The model under review builds one solid part; all positions refer to its coordinate system, in mm. A direction names the side the tool comes from. Coordinates: 2 decimals unless noted, no trailing zeros. Loops run counter-clockwise (first coordinate to the right, second up) from the corner with the lowest first, then second, coordinate; pieces in that order, holes last. Notation, with made-up numbers: M -38.5,65 L 8.5,65 A17 ccw 8.5,80 Z; hole C 11.5,38.25 d1. An arc over 180 degrees is marked long. Use one line per item in the form item = value.
```python
from build123d import *

# Parameters (mm, degrees)
F0_W     = 20
F0_H     = 20
F1_DEPTH = 100
F2_R     = 5
F3_DEPTH = 20.001
F4_R     = 5
F5_DEPTH = 20.001
F6_W     = 22
F6_H     = 20
F6_R     = 5
F7_DEPTH = 10
F8_W     = 30
F8_H     = 20
F8_R     = 5
F9_DEPTH = 10
F10_R    = 9.99999


# Not quite as in the source:
# - a fillet or chamfer is up to 0.001 mm smaller than in the source, because OpenCascade refuses the exact size


with BuildPart() as f1:
    # F0 (on Front) → F1 (new body)
    with BuildSketch(Plane.XZ):
        Rectangle(F0_W, F0_H)
    extrude(amount=F1_DEPTH)

    # F2 (on face) → F3 (cut, through all)
    with BuildSketch(Plane.YZ.offset(10)):
        with Locations((-90, 0)):
            Circle(F2_R)
    extrude(amount=-F3_DEPTH, mode=Mode.SUBTRACT)

    # F4 (on face) → F5 (cut, through all)
    with BuildSketch(Plane.YZ.offset(10)):
        with Locations((-10, 0)):
            Circle(F4_R)
    extrude(amount=-F5_DEPTH, mode=Mode.SUBTRACT)

    # F6 (on face) → F7 (cut)
    with BuildSketch(Plane.YZ.offset(10)):
        with Locations((-11, 0)):
            Rectangle(F6_W, F6_H)
        with Locations((-10, 0)):
            Circle(F6_R, mode=Mode.SUBTRACT)
    extrude(amount=-F7_DEPTH, mode=Mode.SUBTRACT)

    # F8 (on face) → F9 (cut)
    with BuildSketch(Plane(origin=(-10, 0, 0), x_dir=(0, -1, 0), z_dir=(-1, 0, 0))):
        with Locations((85, 0)):
            Rectangle(F8_W, F8_H)
        with Locations((90, 0)):
            Circle(F8_R, mode=Mode.SUBTRACT)
    extrude(amount=-F9_DEPTH, mode=Mode.SUBTRACT)

    # F10 (radius 10 in the source; OpenCascade refuses exactly that, so slightly less here)
    f10_edges = [f1.edges().sort_by_distance(p)[0] for p in [
        (5, -100, 10),
        (5, -100, -10),
        (-5, 0, -10),
        (-5, 0, 10),
    ]]
    fillet(f10_edges, radius=F10_R)


solid = f1.part
```
1. Machinability: for faces 4 (the face through (5, -22, 0)), 5 (the face through (10, -60, 0)), 6 (the face through (-5, -70, 0)), which of the approach directions +Z, -Z, +X, -X, +Y, -Y give a long, thin tool a straight path to every point of the face, cutting with its end or side? Answer none if there is none.
Response values:
face_4 = +Z, -Z, +X, +Y
face_5 = +Z, -Z, +X, +Y, -Y
face_6 = +Z, -Z, -X, -Y
2. Add section D-D (y = -18). State the section outline as (x, z) points, then the cut area to 3 significant figures.
Response values:
outline = M -10,-10 L 0,-10 L 0,10 L -10,10 Z
area = 200 mm^2
3. Add section B-B (z = 2). State the section outline as (x, y) points, then the cut area to 3 significant figures.
Response values:
outline = M -10,-70 L 0,-70 L 0,-85.42 L 10,-85.42 L 10,-22 L 0,-22 L 0,-14.58 L -10,-14.58 Z; M -10,-5.42 L 0,-5.42 L 0,-0.2 L -10,-0.2 Z; M 0,-99.8 L 10,-99.8 L 10,-94.58 L 0,-94.58 Z
area = 1,290 mm^2
4. Wall thickness on line 1 along Z through (x, y) = (7.5, -90); line 2 along Y through (x, z) = (-2, 0.25); line 3 along X through (y, z) = (-16.5, 1): over which ranges is each line inside the solid? List them lowest first. Write a range as from..to.
Response values:
line_1 = -10..-5, 5..10
line_2 = -70..-14.99, -5.01..0
line_3 = -10..0
5. The part is to be moulded in two halves that separate along Z. For faces 1 (the face through (-4.93, -5.23, 1.5)), 2 (the face through (-10, -35, 0)), 3 (the face through (-4.93, -3.01, 7.15)), say which applies: pulls with the +Z half, pulls with the -Z half, needs draft (parallel to the pull), parting line crosses it, or undercut.
Response values:
face_1 = undercut
face_2 = needs draft
face_3 = pulls with the +Z half
6. Insertion check: P1, Ø10, axis at x = -6.5, z = 7.5, coming from the +Y side; P2, Ø9, axis at y = -90, z = 0, coming from the +X side; P3, Ø8, axis at x = -1.5, z = -5.5, coming from the +Y side; P4, Ø5, axis at x = 5, z = -1.5, coming from the +Y side. Each pin has a flat end and moves straight along its axis. Give the tip position at first contact, or say it passes through.
Response values:
P1 = -0.32
P2 = through
P3 = -0.11
P4 = -22
